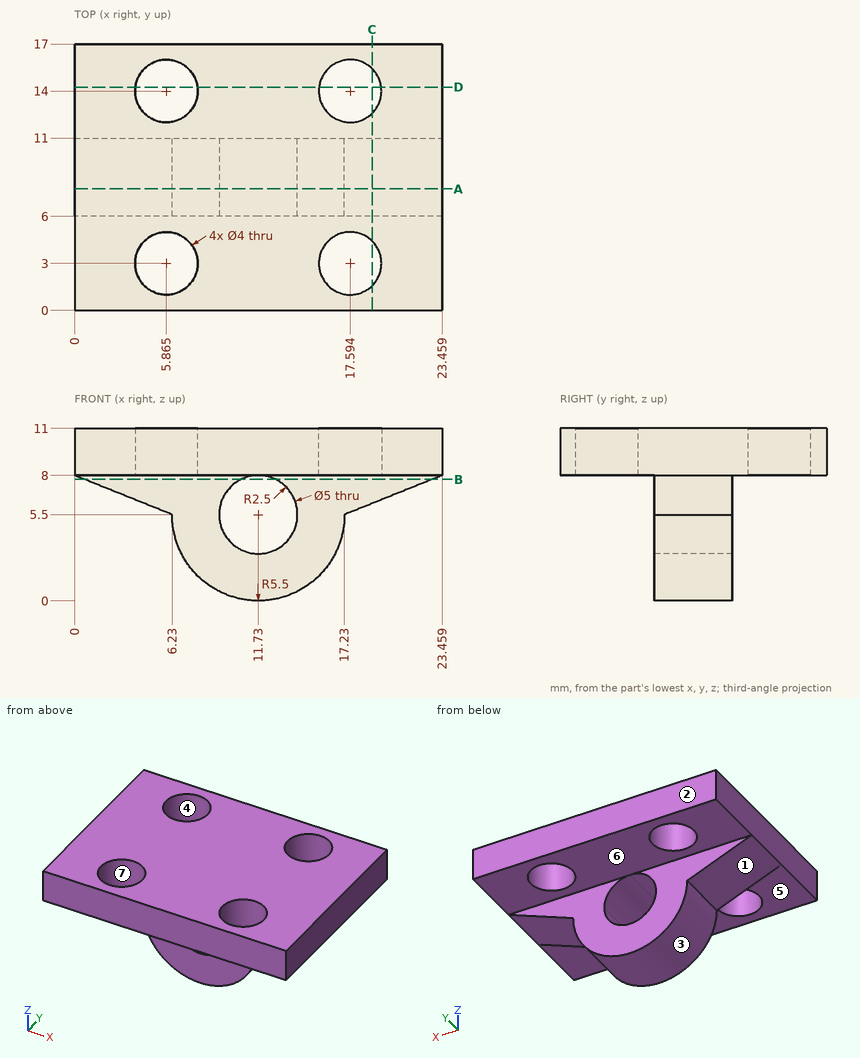
Can you work these out from the drawing? Everything is in mm from the part's minimum corner. A direction names the side the tool comes from. Coordinates: 2 decimals unless noted, no trailing zeros. Order: outer loops, then holes, each group sorted by start corner. A loop starts at its lowest first (then second) coordinate and runs counter-clockwise, first axis right, second up. Notation, with made-up numbers: M 62.5,-23.75 L 74.5,-23.75 A31 ccw 74.5,8.25 Z; hole C 72.5,43.25 d6. An arc over 180 degrees is marked long. Answer as CSV lines item,"result". Start each with the question number.
1. I want a section at A-A, the plane y = 7.75. Write out the boundary of the cut face in (x, z).
2. I want a section at C-C, the plane x = 19. Write out the boundary of the cut face in (y, z).
3. On a 3-axis mill with a long thin cutter (end or side, diameter ignored), from which of +Z, -Z, +X, -X, +Y, -Y can I reach the whole of each face in a straight line? I mean the marked faces 5, 6 and 7. Say none if no direction works.
4. We'd pull the mould along X, two halves only. Please class the marked faces 1, 2, 3 and 4: released by +X, released by -X, zero draft, split by the parting line, or undercut.
5. For pin 1 (4.5 mm diameter, centred on x = 17.59, y = 3, fed in from -Z); pin 2 (4.5 mm diameter, centred on x = 17.59, y = 14, fed in from +Z); pin 3 (5 mm diameter, centred on y = 14.5, z = 4, fed in from +X); pin 4 (5 mm diameter, centred on x = 13, z = 4, fed in from -Y), each with a flat end and sliding along its axis, tell me the tip position at first contact or that it passes through.
6. I want a section at D-D, the plane y = 14.25. Write out the boundary of the cut face in (x, z).
7. I want a section at B-B, the plane z = 7.75. Write out the boundary of the cut face in (x, y), and give its area (3 significant figures).
8. I need wall thicknesses on line 1 (X direction, y = 2.5, z = 10.25); line 2 (Y direction, x = 16.5, z = 10.25) (1 decimal); line 3 (X direction, y = 15.25, z = 8.5) (1 decimal). Which ranges of each line are inside material? Lowest first, please. Write a range as [from, to].
Recorded:
1,outline,"M 0,8 L 6.23,5.5 A5.5 ccw 17.23,5.5 L 23.46,8 L 23.46,11 L 0,11 Z; hole C 11.73,5.5 d5"
2,outline,"M 0,8 L 1.58,8 L 1.58,11 L 0,11 Z; M 4.42,8 L 6,8 L 6,6.21 L 11,6.21 L 11,8 L 12.58,8 L 12.58,11 L 4.42,11 Z; M 15.42,8 L 17,8 L 17,11 L 15.42,11 Z"
3,face 5,"-Z, +X, -X, -Y"
3,face 6,"-Z, +X, -X, +Y"
3,face 7,"+Z, -Z"
4,face 1,"released by -X"
4,face 2,"zero draft"
4,face 3,"split by the parting line"
4,face 4,"undercut"
5,pin 1,"stops at z = 8"
5,pin 2,"stops at z = 11"
5,pin 3,"passes through"
5,pin 4,"stops at y = 6"
6,outline,"M 0,8 L 3.88,8 L 3.88,11 L 0,11 Z; M 7.85,8 L 15.61,8 L 15.61,11 L 7.85,11 Z; M 19.58,8 L 23.46,8 L 23.46,11 L 19.58,11 Z"
7,outline,"M 0.62,6 L 10.64,6 L 10.64,11 L 0.62,11 Z; M 12.82,6 L 22.84,6 L 22.84,11 L 12.82,11 Z"
7,area,"100 mm2"
8,line 1,"x = [0, 3.93], [7.8, 15.66], [19.53, 23.46]"
8,line 2,"y = [0, 1.3], [4.7, 12.3], [15.7, 17]"
8,line 3,"x = [0, 4.3], [7.4, 16], [19.2, 23.5]"
